from build123d import *

# Parameters (mm, degrees)
CHAMFER2_SIZE           = 1
CHAMFER2_SIZE2          = 8.144346428
CUT_EXTRUDE1_DEPTH      = 28.792265111
CUT_EXTRUDE1_DEPTH_BACK = 5
CHAMFER1_SIZE           = 1
CHAMFER3_SIZE           = 0.5
CHAMFER3_SIZE2          = 0.288675135


with BuildPart() as part:
    # Sketch1 → Revolve1 (revolve)
    with BuildSketch(Plane.XY, mode=Mode.PRIVATE) as revolve1_sk:
        Polygon((-15.060768988, 5.5), (-19, 4.805407289), (-19, 0), (-10.35, 0), (-10.35, -0.35), (-8.6, -0.35), (-8.6, -6.85), (-5.6, -6.85), (-5.6, 3.4), (-3, 3.4), (-3, -1.6), (0, -1.6), (0, 5.5), align=None)
    revolve(revolve1_sk.sketch.rotate(Axis((0, -1.6, 0), (0, 1, 0)), 180), axis=Axis((0, -1.6, 0), (0, 1, 0)))

    # Chamfer2
    chamfer2_edges = [part.edges().sort_by_distance(p)[0] for p in [
        (-19, 0, 0),
    ]]
    chamfer2_side = [part.faces().sort_by_distance(p)[0] for p in [
        (-19, 2.402703645, 0),
    ]]
    chamfer(chamfer2_edges, length=CHAMFER2_SIZE, length2=CHAMFER2_SIZE2, reference=chamfer2_side[0])

    # Sketch2 → Cut-Extrude1 (cut, two sides: drawn at the far end of the back side and taken through both)
    with BuildSketch(Plane.XZ.offset(1.6).offset(-CUT_EXTRUDE1_DEPTH_BACK)):
        Polygon((-5.85, 1.85), (-6.6, 1.1), (-6.6, -1.1), (-5.85, -1.85), (-0.35, -1.85), (0.4, -1.1), (0.4, 1.1), (-0.35, 1.85), align=None)
    extrude(amount=CUT_EXTRUDE1_DEPTH + CUT_EXTRUDE1_DEPTH_BACK, mode=Mode.SUBTRACT)

    # Chamfer1
    chamfer1_edges = [part.edges().sort_by_distance(p)[0] for p in [
        (5.6, -6.85, 0),
    ]]
    chamfer(chamfer1_edges, length=CHAMFER1_SIZE)

    # Chamfer3
    chamfer3_edges = [part.edges().sort_by_distance(p)[0] for p in [
        (-8.6, -6.85, 0),
    ]]
    chamfer3_side = [part.faces().sort_by_distance(p)[0] for p in [
        (-8.6, -3.6, 0),
    ]]
    chamfer(chamfer3_edges, length=CHAMFER3_SIZE, length2=CHAMFER3_SIZE2, reference=chamfer3_side[0])


solid = part.part
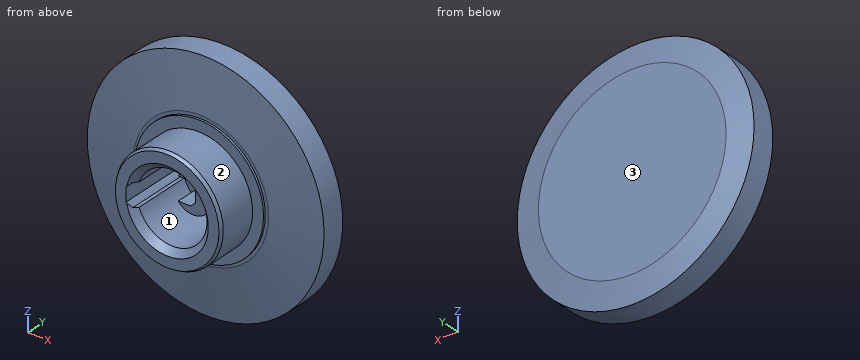
The listing builds one solid part. Answer for the finished solid, in the listing's coordinates (mm). Face numbers are marked on the shaded views. Give positions to 0.01 mm unless a question says otherwise; leave off trailing zeros. Order: outer loops, then holes, each group sorted by start corner. A loop starts at its lowest first (then second) coordinate and runs counter-clockwise, first axis right, second up. Notation, with made-up numbers: (-33.75, 11.25) - (3.25, 11.25) arc R28 cw to (3.25, 36.25) - close; hole circle Ø6 at (-12.75, -2.75). An arc over 180 degrees is marked (long way). One line per item, written item: value. Start each with the question number.
1) Given pin 1 Ø5 at (x, y) = (8, -3) entering from -Z; pin 2 Ø1.5 at (x, y) = (-0.5, -3.5) entering from +Z; pin 3 Ø1 at (x, y) = (-1.5, 1.5) entering from +Z; pin 4 Ø2.5 at (y, z) = (2, 0.5) entering from -X, each flat-ended and moving along its own axis, determine where each tip first touches the part or whether it passes through.
2) A cutting plane is placed at C-C on z = 0. Give the vertices of the cut face in (x, y).
3) A cutting plane is placed at A-A on y = 1.5. Give the vertices of the cut face in (x, z).
4) A cutting plane is placed at D-D on y = -1. Give the vertices of the cut face in (x, z).
5) The mould has two halves that part along X. Classify the marked faces 1, 2 and 3: released by +X, released by -X, zero draft, split by the parting line, or undercut.
6) A cutting plane is placed at B-B on y = -4. Give the vertices of the cut face in (x, z).
7) Find the intervals of material crossed by L1, parallel to Z at x = 0, y = -3; L2, parallel to Z at x = 0, y = -1; L3, parallel to Z at x = -4, y = 3, in increasing order.
Answer sheet:
1. pin 1: stops at z = -6.61
1. pin 2: stops at z = 8.6
1. pin 3: stops at z = 18.97
1. pin 4: stops at x = -19
2. outline: (-19, 1) - (-10.86, 0) - (-10.35, 0) - (-10.35, -0.35) - (-8.6, -0.35) - (-8.6, -6.35) - (-8.31, -6.85) - (-6.6, -6.85) - (-6.6, 3.4) - (0.4, 3.4) - (0.4, -1.6) - (3, -1.6) - (3, 3.4) - (5.6, 3.4) - (5.6, -5.85) - (6.6, -6.85) - (8.31, -6.85) - (8.6, -6.35) - (8.6, -0.35) - (10.35, -0.35) - (10.35, 0) - (10.86, 0) - (19, 1) - (19, 4.81) - (15.06, 5.5) - (-15.06, 5.5) - (-19, 4.81) - close
3. outline: circle Ø38 at (0, 0); (-2.36, -1.85) arc R3 ccw (long way) to (-2.36, 1.85) - (-0.35, 1.85) - (0.4, 1.1) - (0.4, -1.1) - (-0.35, -1.85) - close; hole (-6.6, -1.1) - (-5.85, -1.85) - (-5.29, -1.85) arc R5.6 ccw (long way) to (-5.29, 1.85) - (-5.85, 1.85) - (-6.6, 1.1) - close
4. outline: circle Ø17.2 at (0, 0); (-2.36, -1.85) arc R3 ccw (long way) to (-2.36, 1.85) - (-0.35, 1.85) - (0.4, 1.1) - (0.4, -1.1) - (-0.35, -1.85) - close; hole (-6.6, -1.1) - (-5.85, -1.85) - (-5.29, -1.85) arc R5.6 ccw (long way) to (-5.29, 1.85) - (-5.85, 1.85) - (-6.6, 1.1) - close
5. face 1: undercut
5. face 2: split by the parting line
5. face 3: zero draft
6. outline: circle Ø17.2 at (0, 0); hole (-6.6, -1.1) - (-5.85, -1.85) - (-5.29, -1.85) arc R5.6 ccw (long way) to (-5.29, 1.85) - (-5.85, 1.85) - (-6.6, 1.1) - close
7. L1: z = -8.6 to -5.6, 5.6 to 8.6
7. L2: z = -8.6 to -5.6, -3 to -1.5, 1.5 to 3, 5.6 to 8.6
7. L3: z = -18.57 to -3.92, 3.92 to 18.57
